```python
from build123d import *

# Parameters (mm, degrees)
ESQUISSE1_W                                   = 140
ESQUISSE1_H                                   = 162
BOSS_EXTRU_1_DEPTH                            = 25
TROU_POUR_TARAUDAGE_POUR_TROU_TARAUD_M8_D     = 6.8
TROU_POUR_TARAUDAGE_POUR_TROU_TARAUD_M8_DEPTH = 30
TROU_POUR_TARAUDAGE_POUR_TROU_TARAUD_M8_TIP   = 2.042926105
CHANFREIN1_SIZE                               = 35
CONG_3_R                                      = 6
ESQUISSE15_R                                  = 12
ENL_V_MAT_EXTRU_4_DEPTH                       = 22
ESQUISSE16_R                                  = 11
ENL_V_MAT_EXTRU_5_DEPTH                       = 110.293183685
TROU_POUR_TARAUDAGE_POUR_TROU_TARAUD_M4_D     = 3.3
TROU_POUR_TARAUDAGE_POUR_TROU_TARAUD_M4_DEPTH = 15
TROU_POUR_TARAUDAGE_POUR_TROU_TARAUD_M4_TIP   = 0.991420021
ESQUISSE41_R                                  = 25.5
ENL_V_MAT_EXTRU_15_DEPTH                      = 5
TROU_POUR_TARAUDAGE_POUR_TROU_TARAUD_M6_D     = 5
TROU_POUR_TARAUDAGE_POUR_TROU_TARAUD_M6_DEPTH = 12
TROU_POUR_TARAUDAGE_POUR_TROU_TARAUD_M6_TIP   = 1.502151548
RAINURE_DE_CHAMBRAGE_POUR_VIS_T_TE_HEX_DEPTH  = 25
RAINURE_START                                 = 19.6
RAINURE_DE_CHAMBRAGE_POUR_VIS_T_TE_3_DEPTH    = 5.4


# Read off the part's stored shape, not the designer's step: Rainure de chambrage pour vis à tête hexagonale M52
with BuildPart() as part:
    # Esquisse1 → Boss.-Extru.1 (new body)
    with BuildSketch(Plane.XY):
        Rectangle(ESQUISSE1_W, ESQUISSE1_H)
    extrude(amount=BOSS_EXTRU_1_DEPTH)

    # Trou pour taraudage pour trou taraudé M81
    with Locations(Plane(origin=(0, 81, 0), x_dir=(1, 0, 0), z_dir=(0, 1, 0))):
        with Locations((-57.5, -12.5), (57.5, -12.5)):
            Hole(TROU_POUR_TARAUDAGE_POUR_TROU_TARAUD_M8_D / 2, depth=TROU_POUR_TARAUDAGE_POUR_TROU_TARAUD_M8_DEPTH)
            with Locations((0, 0, -(TROU_POUR_TARAUDAGE_POUR_TROU_TARAUD_M8_DEPTH + TROU_POUR_TARAUDAGE_POUR_TROU_TARAUD_M8_TIP / 2))):  # 118° drill point
                Cone(0, TROU_POUR_TARAUDAGE_POUR_TROU_TARAUD_M8_D / 2, TROU_POUR_TARAUDAGE_POUR_TROU_TARAUD_M8_TIP, mode=Mode.SUBTRACT)

    # Chanfrein1
    chanfrein1_edges = [part.edges().sort_by_distance(p)[0] for p in [
        (70, -81, 12.5),
        (-70, -81, 12.5),
    ]]
    chamfer(chanfrein1_edges, length=CHANFREIN1_SIZE)

    # Congé3
    cong_3_edges = [part.edges().sort_by_distance(p)[0] for p in [
        (35, -81, 12.5),
        (-35, -81, 12.5),
        (-70, -46, 12.5),
        (70, -46, 12.5),
    ]]
    fillet(cong_3_edges, radius=CONG_3_R)

    # Esquisse15 → Enlèv. mat.-Extru.4 (cut)
    with BuildSketch(Plane(origin=(0, 0, 0), x_dir=(-1, 0, 0), z_dir=(0, 0, -1))):
        with Locations((0, -45.83)):
            Circle(ESQUISSE15_R)
    extrude(amount=-ENL_V_MAT_EXTRU_4_DEPTH, mode=Mode.SUBTRACT)

    # Esquisse16 → Enlèv. mat.-Extru.5 (cut, through all)
    with BuildSketch(Plane(origin=(0, 0, 22), x_dir=(-1, 0, 0), z_dir=(0, 0, -1))):
        with Locations((0, -45.83)):
            Circle(ESQUISSE16_R)
    extrude(amount=-ENL_V_MAT_EXTRU_5_DEPTH, mode=Mode.SUBTRACT)

    # Trou pour taraudage pour trou taraudé M41
    with Locations(Plane(origin=(0, 0, 0), x_dir=(-1, 0, 0), z_dir=(0, 0, -1))):
        with Locations((-65, -35.83), (-51, -35.83)):
            Hole(TROU_POUR_TARAUDAGE_POUR_TROU_TARAUD_M4_D / 2, depth=TROU_POUR_TARAUDAGE_POUR_TROU_TARAUD_M4_DEPTH)
            with Locations((0, 0, -(TROU_POUR_TARAUDAGE_POUR_TROU_TARAUD_M4_DEPTH + TROU_POUR_TARAUDAGE_POUR_TROU_TARAUD_M4_TIP / 2))):  # 118° drill point
                Cone(0, TROU_POUR_TARAUDAGE_POUR_TROU_TARAUD_M4_D / 2, TROU_POUR_TARAUDAGE_POUR_TROU_TARAUD_M4_TIP, mode=Mode.SUBTRACT)

    # Esquisse41 → Enlèv. mat.-Extru.15 (cut)
    with BuildSketch(Plane(origin=(0, 0, 0), x_dir=(-1, 0, 0), z_dir=(0, 0, -1))):
        with Locations((0, -45.83)):
            Circle(ESQUISSE41_R)
    extrude(amount=-ENL_V_MAT_EXTRU_15_DEPTH, mode=Mode.SUBTRACT)

    # Trou pour taraudage pour trou taraudé M61
    with Locations(Plane(origin=(0, 0, 5), x_dir=(-1, 0, 0), z_dir=(0, 0, -1))):
        with Locations((12.727922061, -33.102077939), (-12.727922061, -58.557922061), (-12.727922061, -33.102077939), (12.727922061, -58.557922061)):
            Hole(TROU_POUR_TARAUDAGE_POUR_TROU_TARAUD_M6_D / 2, depth=TROU_POUR_TARAUDAGE_POUR_TROU_TARAUD_M6_DEPTH)
            with Locations((0, 0, -(TROU_POUR_TARAUDAGE_POUR_TROU_TARAUD_M6_DEPTH + TROU_POUR_TARAUDAGE_POUR_TROU_TARAUD_M6_TIP / 2))):  # 118° drill point
                Cone(0, TROU_POUR_TARAUDAGE_POUR_TROU_TARAUD_M6_D / 2, TROU_POUR_TARAUDAGE_POUR_TROU_TARAUD_M6_TIP, mode=Mode.SUBTRACT)

    # Rainure de chambrage pour vis _ t_te 2 → Rainure de chambrage pour vis à tête hexagonale M52 (cut)
    with BuildSketch(Plane.XY):
        with BuildLine():
            Line((-50.72, -24.484553863), (-50.72, -1.784553863))
            ThreePointArc((-50.72, -1.784553863), (-53.37, 0.865446137), (-56.02, -1.784553863))
            Line((-56.02, -1.784553863), (-56.02, -24.484553863))
            ThreePointArc((-56.02, -24.484553863), (-53.37, -27.134553863), (-50.72, -24.484553863))
        make_face()
        with BuildLine():
            Line((-50.72, 22.655446137), (-50.72, 45.355446137))
            ThreePointArc((-50.72, 45.355446137), (-53.37, 48.005446137), (-56.02, 45.355446137))
            Line((-56.02, 45.355446137), (-56.02, 22.655446137))
            ThreePointArc((-56.02, 22.655446137), (-53.37, 20.005446137), (-50.72, 22.655446137))
        make_face()
        with BuildLine():
            Line((-8.85, 45.355446137), (-8.85, 22.655446137))
            ThreePointArc((-8.85, 22.655446137), (-6.2, 20.005446137), (-3.55, 22.655446137))
            Line((-3.55, 22.655446137), (-3.55, 45.355446137))
            ThreePointArc((-3.55, 45.355446137), (-6.2, 48.005446137), (-8.85, 45.355446137))
        make_face()
    extrude(amount=RAINURE_DE_CHAMBRAGE_POUR_VIS_T_TE_HEX_DEPTH, mode=Mode.SUBTRACT)

    # Rainure de chambrage pour vis _ t_te 3 o → Rainure de chambrage pour vis _ t_te 3 (cut)
    # profile 1 of 3: a face of its own
    with BuildSketch(Plane.XY.offset(RAINURE_START)):
        with BuildLine():
            Line((-58.37, -1.784553863), (-58.37, -24.484553863))
            ThreePointArc((-58.37, -24.484553863), (-53.37, -29.484553863), (-48.37, -24.484553863))
            Line((-48.37, -24.484553863), (-48.37, -1.784553863))
            ThreePointArc((-48.37, -1.784553863), (-53.37, 3.215446137), (-58.37, -1.784553863))
        make_face()
        with BuildLine():
            ThreePointArc((-56.02, -1.784553863), (-53.37, 0.865446137), (-50.72, -1.784553863))
            Line((-50.72, -1.784553863), (-50.72, -24.484553863))
            ThreePointArc((-50.72, -24.484553863), (-53.37, -27.134553863), (-56.02, -24.484553863))
            Line((-56.02, -24.484553863), (-56.02, -1.784553863))
        make_face(mode=Mode.SUBTRACT)
    # profile 2 of 3: a face of its own
    with BuildSketch(Plane.XY.offset(RAINURE_START)):
        with BuildLine():
            Line((-48.37, 22.655446137), (-48.37, 45.355446137))
            ThreePointArc((-48.37, 45.355446137), (-53.37, 50.355446137), (-58.37, 45.355446137))
            Line((-58.37, 45.355446137), (-58.37, 22.655446137))
            ThreePointArc((-58.37, 22.655446137), (-53.37, 17.655446137), (-48.37, 22.655446137))
        make_face()
        with BuildLine():
            ThreePointArc((-56.02, 45.355446137), (-53.37, 48.005446137), (-50.72, 45.355446137))
            Line((-50.72, 45.355446137), (-50.72, 22.655446137))
            ThreePointArc((-50.72, 22.655446137), (-53.37, 20.005446137), (-56.02, 22.655446137))
            Line((-56.02, 22.655446137), (-56.02, 45.355446137))
        make_face(mode=Mode.SUBTRACT)
    # profile 3 of 3: a face of its own
    with BuildSketch(Plane.XY.offset(RAINURE_START)):
        with BuildLine():
            Line((-11.2, 45.355446137), (-11.2, 22.655446137))
            ThreePointArc((-11.2, 22.655446137), (-6.2, 17.655446137), (-1.2, 22.655446137))
            Line((-1.2, 22.655446137), (-1.2, 45.355446137))
            ThreePointArc((-1.2, 45.355446137), (-6.2, 50.355446137), (-11.2, 45.355446137))
        make_face()
        with BuildLine():
            ThreePointArc((-3.55, 22.655446137), (-6.2, 20.005446137), (-8.85, 22.655446137))
            Line((-8.85, 22.655446137), (-8.85, 45.355446137))
            ThreePointArc((-8.85, 45.355446137), (-6.2, 48.005446137), (-3.55, 45.355446137))
            Line((-3.55, 45.355446137), (-3.55, 22.655446137))
        make_face(mode=Mode.SUBTRACT)
    extrude(amount=RAINURE_DE_CHAMBRAGE_POUR_VIS_T_TE_3_DEPTH, mode=Mode.SUBTRACT)


solid = part.part
```
Here's how the part is built. I have some questions about the finished solid (model axes, mm). A direction names the side the tool comes from. Give positions to 0.01 mm unless a question says otherwise; leave off trailing zeros. Order: outer loops, then holes, each group sorted by start corner. A loop starts at its lowest first (then second) coordinate and runs counter-clockwise, first axis right, second up. Notation, with made-up numbers: (-9.5, 20.5) - (42.5, 20.5) arc R14 cw to (42.5, 37.5) - close; hole circle Ø3 at (13.25, -27). An arc over 180 degrees is marked (long way). Answer as a JSON object with one key per item and string values. Group by question number.
Item 1: If we section it at A-A on y = -7: Please give me the cut outline in (x, z), and give its area (3 significant figures).
Item 2: If we section it at B-B on x = 40: Please give me the cut outline in (y, z), and give its area (4 significant figures).
Item 3: Which directions (+Z, -Z, +X, -X, +Y, -Y) give clear straight access to the entire face, cutting with the end or side of a thin tool? Please do faces 5 (the flat face through (-57, -13, 19.6)), 6 (the cylindrical face through (-53.312, 48.005, 9.663)), 7 (the cylindrical face through (12.186, -35.543, 11.084)).
Item 4: Please list where these lines run through material, in increasing order: probe 1 along X at (y, z) = (73.25, 12.5); probe 2 along X at (y, z) = (-33, 10.75); probe 3 along X at (y, z) = (-35.83, 4.25).
Item 5: For P1, Ø10, axis at x = -38, y = 41.5, coming from the -Z side; P2, Ø6, axis at x = 57.5, z = 12.5, coming from the -Y side; P3, Ø3, axis at x = -1, y = -28, coming from the -Z side; P4, Ø5, axis at x = -8.5, y = 35.5, coming from the +Z side, each with a flat end and sliding along its axis, tell me the tip position at first contact or that it passes through.
Item 6: If we section it at C-C on x = -43: Please give me the cut outline in (y, z), and give its area (3 significant figures).
Item 7: If we mould it in two halves opening along Z, with no side actions, what happens to faces 1 (the cylindrical face through (-34.84, -80.53, 12.68)), 2 (the flat face through (-10, 34, 19.6)), 3 (the cylindrical face through (54.36, 65.79, 13.8)), 4 (the flat face through (-1, 19, 0))? For each: pulls with the +Z half, pulls with the -Z half, needs draft (parallel to the pull), parting line crosses it, or undercut.
Result set:
{
 "1": {"outline": "(-70, 0) - (-56.02, 0) - (-56.02, 19.6) - (-58.37, 19.6) - (-58.37, 25) - (-70, 25) - close; (-50.72, 0) - (70, 0) - (70, 25) - (-48.37, 25) - (-48.37, 19.6) - (-50.72, 19.6) - close", "area": "3,340 mm²"},
 "2": {"outline": "(-76, 0) - (81, 0) - (81, 25) - (-76, 25) - close", "area": "3,925 mm²"},
 "3": {"face 5": "+Z", "face 6": "+Z, -Z", "face 7": "-Z"},
 "4": {"probe 1": "-70 to -60.9, -54.1 to 54.1, 60.9 to 70", "probe 2": "-70 to -15.23, -10.23 to 10.23, 15.23 to 70", "probe 3": "-70 to -23.46, 23.46 to 49.35, 52.65 to 63.35, 66.65 to 70"},
 "5": {"P1": "z = 0", "P2": "y = -61.5", "P3": "z = 5", "P4": "z = 19.6"},
 "6": {"outline": "(-73, 0) - (81, 0) - (81, 25) - (-73, 25) - close", "area": "3,850 mm²"},
 "7": {"face 1": "needs draft", "face 2": "pulls with the +Z half", "face 3": "undercut", "face 4": "pulls with the -Z half"}
}
